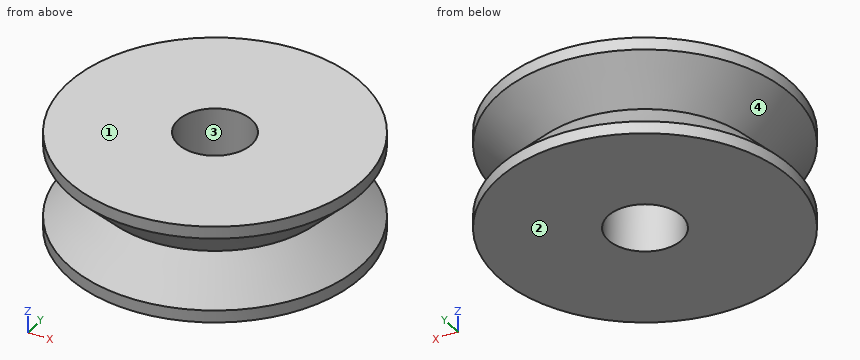
```python
from build123d import *

# Parameters (mm, degrees)
SKETCH1_R           = 6
SKETCH1_R_2         = 1.5
BOSS_EXTRUDE1_DEPTH = 2
CHAMFER1_SIZE       = 1.5
SKETCH2_R           = 6
SKETCH2_R_2         = 1.5
BOSS_EXTRUDE2_DEPTH = 2
CHAMFER2_SIZE       = 1.5


with BuildPart() as part:
    # Sketch1 → Boss-Extrude1 (new body)
    with BuildSketch(Plane.XY):
        Circle(SKETCH1_R)
        Circle(SKETCH1_R_2, mode=Mode.SUBTRACT)
    extrude(amount=BOSS_EXTRUDE1_DEPTH)

    # Chamfer1
    chamfer1_edges = [part.edges().sort_by_distance(p)[0] for p in [
        (-6, 0, 2),
    ]]
    chamfer(chamfer1_edges, length=CHAMFER1_SIZE)

    # Sketch2 → Boss-Extrude2 (add)
    with BuildSketch(Plane.XY.offset(2)):
        Circle(SKETCH2_R)
        Circle(SKETCH2_R_2, mode=Mode.SUBTRACT)
    extrude(amount=BOSS_EXTRUDE2_DEPTH)

    # Chamfer2
    chamfer2_edges = [part.edges().sort_by_distance(p)[0] for p in [
        (-6, 0, 2),
    ]]
    chamfer(chamfer2_edges, length=CHAMFER2_SIZE - 0.0001)  # a hair under: the kernel refuses the full size


solid = part.part
```
CAD build for the part. Positions are in the model's coordinates, mm. Face numbers are marked on the shaded views. Coordinates: 2 decimals unless noted, no trailing zeros. Order: outer loops, then holes, each group sorted by start corner. A loop starts at its lowest first (then second) coordinate and runs counter-clockwise, first axis right, second up. Notation, with made-up numbers: (61.5, 87) -> (82.5, 87) arc R8 cw to (82.5, 93) -> close; hole circle Ø1 at (87, 28). An arc over 180 degrees is marked (long way). Use one line per item in the form item = value. Start each with the question number.
1) Pull direction Z, two halves, no side cores. Call the marked faces 1, 2, 3 and 4: +Z half, -Z half, draft (parallel to the pull), parting line (faces both ways), or undercut.
2) Band-saw the part on C-C on z = 1.2. Give the cut face in (x, y).
3) Band-saw the part on D-D on z = 3.65. Give the cut face in (x, y), then the cut area to 3 significant figures.
4) Drop a flat-ended pin along its axis: pin 1 (2 mm diameter, centred on y = -1.5, z = 3.5, fed in from -X). Give the stop position or say it passes through.
5) Drill centre lines: L1, parallel to Y at x = 0, z = 1.5; L2, parallel to Z at x = 2, y = -5.5; L3, parallel to Z at x = 3.75, y = 4. Where is each one in solid material? Low to high. Write a range as [from, to].
Entries:
q1.face_1 = +Z half
q1.face_2 = -Z half
q1.face_3 = draft
q1.face_4 = undercut
q2.outline = circle Ø10.6 at (0, 0); hole circle Ø3 at (0, 0)
q3.outline = circle Ø12 at (0, 0); hole circle Ø3 at (0, 0)
q3.area = 106 mm2
q4.pin_1 = -5.98
q5.L1 = [-5, -1.5], [1.5, 5]
q5.L2 = [0, 0.65], [3.35, 4]
q5.L3 = [0, 1.02], [2.98, 4]
